Can you work these out from the model? Positions are in its coordinate system, mm. A direction names the side the tool comes from. Give positions to 0.01 mm unless a question says otherwise; leave off trailing zeros. Write each loop counter-clockwise with the first axis right and the second up, starting at its lowest first coordinate (ties: lowest second). Pieces come first, ordered by that corner, then holes.
```python
from build123d import *
from OCP.BRepFilletAPI import BRepFilletAPI_MakeChamfer

# Parameters (mm, degrees)
SKETCH1_W           = 39.751
SKETCH1_H           = 12.7
BOSS_EXTRUDE1_DEPTH = 1.8288
SKETCH2_W           = 29.0322
SKETCH2_H           = 12.7
BOSS_EXTRUDE2_DEPTH = 19.812
SKETCH3_W           = 28.956
SKETCH3_H           = 12.7
BOSS_EXTRUDE3_DEPTH = 7.366
SKETCH4_R           = 5.842
BOSS_EXTRUDE4_DEPTH = 1.27
SKETCH5_R           = 2.921
BOSS_EXTRUDE5_DEPTH = 4.064
SKETCH6_W           = 3.81
SKETCH6_H           = 7.62
BOSS_EXTRUDE6_DEPTH = 6.35
CHAMFER1_SIZE       = 5.08
CHAMFER1_SIZE2      = 0.508
FILLET1_R           = 1.27
CUT_EXTRUDE1_REACH  = 49.849
SKETCH7_R           = 2.54
FILLET2_R           = 0.254
FILLET3_R           = 0.508


with BuildPart() as part:
    # Sketch1 → Boss-Extrude1 (new body)
    with BuildSketch(Plane.XY):
        with Locations((19.8755, 6.35)):
            Rectangle(SKETCH1_W, SKETCH1_H)
    extrude(amount=BOSS_EXTRUDE1_DEPTH)

    # Sketch2 → Boss-Extrude2 (add)
    with BuildSketch(Plane.XY.offset(1.8288)):
        with Locations((19.8755, 6.35)):
            Rectangle(SKETCH2_W, SKETCH2_H)
    extrude(amount=BOSS_EXTRUDE2_DEPTH)

    # Sketch3 → Boss-Extrude3 (add)
    with BuildSketch(Plane(origin=(0, 0, 0), x_dir=(-1, 0, 0), z_dir=(0, 0, -1))):
        with Locations((-19.8755, 6.35)):
            Rectangle(SKETCH3_W, SKETCH3_H)
    extrude(amount=BOSS_EXTRUDE3_DEPTH)

    # Sketch4 → Boss-Extrude4 (add)
    with BuildSketch(Plane(origin=(0, 0, -7.366), x_dir=(-1, 0, 0), z_dir=(0, 0, -1))):
        with Locations((-27.2415, 6.35)):
            Circle(SKETCH4_R)
    extrude(amount=BOSS_EXTRUDE4_DEPTH)

    # Sketch5 → Boss-Extrude5 (add)
    with BuildSketch(Plane(origin=(0, 0, -8.636), x_dir=(-1, 0, 0), z_dir=(0, 0, -1))):
        with Locations((-27.2415, 6.35)):
            Circle(SKETCH5_R)
    extrude(amount=BOSS_EXTRUDE5_DEPTH)

    # Sketch6 → Boss-Extrude6 (add)
    with BuildSketch(Plane(origin=(34.3916, 0, 0), x_dir=(0, 0, -1), z_dir=(1, 0, 0))):
        with Locations((-19.2278, 6.35)):
            Rectangle(SKETCH6_W, SKETCH6_H)
    extrude(amount=BOSS_EXTRUDE6_DEPTH)

    # Chamfer1: one chamfer whose edges measure the first distance from different faces: ONE call of the kernel's chamfer builder (chamfer() names one face for all edges)
    chamfer1_edges_1 = [part.edges().sort_by_distance(p)[0] for p in [
        (40.7416, 6.35, 21.1328),
    ]]
    chamfer1_side_1 = [part.faces().sort_by_distance(p)[0] for p in [
        (37.5666, 6.35, 21.1328),
    ]]
    chamfer1_edges_2 = [part.edges().sort_by_distance(p)[0] for p in [
        (40.7416, 2.54, 19.2278),
    ]]
    chamfer1_side_2 = [part.faces().sort_by_distance(p)[0] for p in [
        (37.5666, 2.54, 19.2278),
    ]]
    chamfer1_edges_3 = [part.edges().sort_by_distance(p)[0] for p in [
        (40.7416, 6.35, 17.3228),
    ]]
    chamfer1_side_3 = [part.faces().sort_by_distance(p)[0] for p in [
        (37.5666, 6.35, 17.3228),
    ]]
    chamfer1_edges_4 = [part.edges().sort_by_distance(p)[0] for p in [
        (40.7416, 10.16, 19.2278),
    ]]
    chamfer1_side_4 = [part.faces().sort_by_distance(p)[0] for p in [
        (37.5666, 10.16, 19.2278),
    ]]
    chamfer1 = BRepFilletAPI_MakeChamfer(part.part.solid().wrapped)
    for e in chamfer1_edges_1:
        chamfer1.Add(CHAMFER1_SIZE, CHAMFER1_SIZE2, e.wrapped, chamfer1_side_1[0].wrapped)  # the first distance lies on this face
    for e in chamfer1_edges_2:
        chamfer1.Add(CHAMFER1_SIZE, CHAMFER1_SIZE2, e.wrapped, chamfer1_side_2[0].wrapped)  # the first distance lies on this face
    for e in chamfer1_edges_3:
        chamfer1.Add(CHAMFER1_SIZE, CHAMFER1_SIZE2, e.wrapped, chamfer1_side_3[0].wrapped)  # the first distance lies on this face
    for e in chamfer1_edges_4:
        chamfer1.Add(CHAMFER1_SIZE, CHAMFER1_SIZE2, e.wrapped, chamfer1_side_4[0].wrapped)  # the first distance lies on this face
    add(Compound.cast(chamfer1.Shape()), mode=Mode.REPLACE)

    # Fillet1
    fillet1_edges = [part.edges().sort_by_distance(p)[0] for p in [
        (5.3594, 12.7, 11.7348),
        (5.3594, 0, 11.7348),
        (34.3916, 0, 11.7348),
        (34.3916, 12.7, 11.7348),
        (34.3535, 12.7, -3.683),
        (34.3535, 0, -3.683),
        (5.3975, 0, -3.683),
        (5.3975, 12.7, -3.683),
        (0, 0, 0.9144),
        (39.751, 0, 0.9144),
        (39.751, 12.7, 0.9144),
        (0, 12.7, 0.9144),
    ]]
    fillet(fillet1_edges, radius=FILLET1_R)

    # Sketch7 → Cut-Extrude1 (cut, up to next)
    with BuildSketch(Plane(origin=(0, 0, 0), x_dir=(-1, 0, 0), z_dir=(0, 0, -1)), mode=Mode.PRIVATE) as cut_extrude1_sk1:
        with Locations((-37.4015, 6.35)):
            Circle(SKETCH7_R)
    cut_extrude1_tool1 = extrude(cut_extrude1_sk1.sketch, amount=-CUT_EXTRUDE1_REACH, mode=Mode.PRIVATE) & part.part
    # Sketch7 → Cut-Extrude1 (cut, up to next)
    with BuildSketch(Plane(origin=(0, 0, 0), x_dir=(-1, 0, 0), z_dir=(0, 0, -1)), mode=Mode.PRIVATE) as cut_extrude1_sk2:
        with Locations((-2.3495, 6.35)):
            Circle(SKETCH7_R)
    cut_extrude1_tool2 = extrude(cut_extrude1_sk2.sketch, amount=-CUT_EXTRUDE1_REACH, mode=Mode.PRIVATE) & part.part
    add(cut_extrude1_tool1.solids().sort_by_distance((37.4015, 6.35, 0))[0], mode=Mode.SUBTRACT)
    add(cut_extrude1_tool2.solids().sort_by_distance((2.3495, 6.35, 0))[0], mode=Mode.SUBTRACT)

    # Fillet2
    fillet2_edges = [part.edges().sort_by_distance(p)[0] for p in [
        (39.751, 7.315116444, 0.9144),
        (39.751, 5.384883556, 0.9144),
        (0, 7.315116444, 0.9144),
        (0, 5.384883556, 0.9144),
    ]]
    fillet(fillet2_edges, radius=FILLET2_R)

    # Fillet3
    fillet3_edges = [part.edges().sort_by_distance(p)[0] for p in [
        (33.0835, 6.35, -8.636),
    ]]
    fillet(fillet3_edges, radius=FILLET3_R)


solid = part.part
```
1) If we mould it in two halves opening along Y, with no side actions, what happens to faces 6 (the face through (33.97, 0.36, -3.73)), 7 (the face through (4.888, 6.436, 0.902)), 8 (the face through (34.863, 6.264, 0.902)), 9 (the face through (25, 4, -8.636))? For each: +Y half, -Y half, draft (parallel to the pull), parting line (faces both ways), or undercut.
Values follow:
face 6: -Y half
face 7: undercut
face 8: undercut
face 9: draft
2) Suppose I cut it at B-B on z = -6.5. Write out the boundary of the cut face in (x, y), plus the area to 3 significant figures.
Values follow:
outline: (5.4, 1.27) arc R1.27 ccw to (6.67, 0) - (33.08, 0) arc R1.27 ccw to (34.35, 1.27) - (34.35, 11.43) arc R1.27 ccw to (33.08, 12.7) - (6.67, 12.7) arc R1.27 ccw to (5.4, 11.43) - close
area: 366 mm2
3) Suppose I cut it at C-C on y = 6.35. Write out the boundary of the cut face in (x, z).
Values follow:
outline: (4.89, 0) - (5.4, 0) - (5.4, -7.37) - (21.4, -7.37) - (21.4, -8.13) arc R0.51 ccw to (21.91, -8.64) - (24.32, -8.64) - (24.32, -12.7) - (30.16, -12.7) - (30.16, -8.64) - (32.58, -8.64) arc R0.51 ccw to (33.08, -8.13) - (33.08, -7.37) - (34.35, -7.37) - (34.35, 0) - (34.86, 0) - (34.86, 1.83) - (34.39, 1.83) - (34.39, 17.32) - (35.66, 17.32) - (40.74, 17.83) - (40.74, 20.62) - (35.66, 21.13) - (34.39, 21.13) - (34.39, 21.64) - (5.36, 21.64) - (5.36, 1.83) - (4.89, 1.83) - close
4) Suppose I cut it at D-D on x = 8.5. Write out the boundary of the cut face in (y, z).
Values follow:
outline: (0, -7.37) - (12.7, -7.37) - (12.7, 21.64) - (0, 21.64) - close
5) Please list where these lines run through material, in increasing order: L1, parallel to Z at x = 12, y = 11; L2, parallel to Z at x = 37, y = 2.5; L3, parallel to X at y = 7, z = 14.
Values follow:
L1: z = -7.37 to 21.64
L2: z = 0 to 1.83
L3: x = 5.36 to 34.39
6) Suppose I cut it at A-A on x = 37. Write out the boundary of the cut face in (y, z).
Values follow:
outline: (0, 0) - (3.84, 0) - (3.84, 1.83) - (0, 1.83) - close; (2.67, 17.46) - (10.03, 17.46) - (10.03, 21) - (2.67, 21) - close; (8.86, 0) - (12.7, 0) - (12.7, 1.83) - (8.86, 1.83) - close
7) For faces 1 (the face through (5.78, 12.34, -3.73)), 2 (the face through (38.237, 2.798, 19.254)), 3 (the face through (27.622, 9.246, -10.64)), 4 (the face through (5.397, 6, -4)), 5 (the face through (34.03, 12.32, 11.87)), which set-ups out of +Z, -Z, +X, -X, +Y, -Y let a thin tool reach every point of the face, with its end or its side?
Values follow:
face 1: -Z, -X, +Y
face 2: +Z, +X, -Y
face 3: -Z
face 4: -Z, -X, +Y, -Y
face 5: +Z, +X, +Y
8) For pin 1 Ø5 at (y, z) = (1.5, 14.5) entering from +X; pin 2 Ø1 at (x, y) = (23, 5) entering from -Z; pin 3 Ø4.5 at (x, y) = (37.4, 6.35) entering from -Z, each with a flat end and sliding along its axis, tell me the tip position at first contact or that it passes through.
Values follow:
pin 1: stops at x = 34.39
pin 2: stops at z = -8.64
pin 3: stops at z = 17.32
